Model file for the job. Use its own axes, mm. A direction names the side the tool comes from. Round coordinates to 2 decimals unless told otherwise and drop trailing zeros. Loops run counter-clockwise (first coordinate to the right, second up) from the corner with the lowest first, then second, coordinate; pieces in that order, holes last.
from build123d import *

# Parameters (mm, degrees)
SKETCH2_W                = 20
SKETCH2_H                = 64
BOSS_EXTRUDE1_DEPTH      = 30
SKETCH3_R                = 4
CUT_EXTRUDE1_DEPTH       = 20
SKETCH4_R                = 2.5
CUT_EXTRUDE2_DEPTH       = 10
FILLET1_R                = 10
BOSS_EXTRUDE2_DEPTH      = 20
BOSS_EXTRUDE2_DEPTH_BACK = 30
SKETCH5_W                = 2
SKETCH5_H                = 30
CUT_EXTRUDE3_REACH       = 55.161
SKETCH6_R                = 2.5
SKETCH6_W                = 10
SKETCH6_H                = 20
SKETCH6_W_2              = 20
SKETCH6_H_2              = 10
FILLET2_R                = 5
SKETCH7_W                = 21
SKETCH7_H                = 6
CUT_EXTRUDE4_DEPTH       = 10


with BuildPart() as part:
    # Sketch2 → Boss-Extrude1 (new body)
    with BuildSketch(Plane(origin=(0, 0, 0), x_dir=(1, 0, 0), z_dir=(0, 1, 0))):
        with Locations((6.47761194, -8.23880597)):
            Rectangle(SKETCH2_W, SKETCH2_H)
    extrude(amount=BOSS_EXTRUDE1_DEPTH)

    # Sketch3 → Cut-Extrude1 (cut)
    with BuildSketch(Plane(origin=(0, 30, 0), x_dir=(1, 0, 0), z_dir=(0, 1, 0))):
        with Locations(Location((6.47761194, 13.76119403, 0), (0, 0, 270))):
            Circle(SKETCH3_R)
        with Locations(Location((6.47761194, -30.23880597, 0), (0, 0, 270))):
            Circle(SKETCH3_R)
    extrude(amount=-CUT_EXTRUDE1_DEPTH, mode=Mode.SUBTRACT)

    # Sketch4 → Cut-Extrude2 (cut)
    with BuildSketch(Plane.ZY.offset(3.52238806)):
        with BuildLine():
            Line((17.415034126, 30.126407987), (14.795699792, 30.126407987))
            Line((14.795699792, 30.126407987), (14.949961333, 28.969446425))
            ThreePointArc((14.949961333, 28.969446425), (16.17927412, 22.186618473), (17.347611009, 28.980215007))
            Line((17.347611009, 28.980215007), (17.415034126, 30.126407987))
        make_face()
        with Locations((16.163554702, 25.686583173)):
            Circle(SKETCH4_R, mode=Mode.SUBTRACT)
    extrude(amount=-CUT_EXTRUDE2_DEPTH, mode=Mode.SUBTRACT)

    # Fillet1
    fillet1_edges = [part.edges().sort_by_distance(p)[0] for p in [
        (-3.52238806, 15, -23.76119403),
        (16.47761194, 15, -23.76119403),
        (16.47761194, 15, 40.23880597),
        (-3.52238806, 15, 40.23880597),
    ]]
    fillet(fillet1_edges, radius=FILLET1_R - 0.0001)  # a hair under: the kernel refuses the full size

    # Sketch5 → Boss-Extrude2 (add, two sides: drawn at the far end of the back side and taken through both)
    with BuildSketch(Plane.ZY.offset(3.52238806).offset(-BOSS_EXTRUDE2_DEPTH_BACK)):
        with Locations((6.23880597, 15)):
            Rectangle(SKETCH5_W, SKETCH5_H)
    extrude(amount=BOSS_EXTRUDE2_DEPTH + BOSS_EXTRUDE2_DEPTH_BACK)

    # Sketch6 → Cut-Extrude3 (cut, up to next)
    with BuildSketch(Plane(origin=(0, 0, 5.23880597), x_dir=(-1, 0, 0), z_dir=(0, 0, -1)), mode=Mode.PRIVATE) as cut_extrude3_sk1:
        with Locations((-21.47761194, 5)):
            Circle(SKETCH6_R)
    cut_extrude3_tool1 = extrude(cut_extrude3_sk1.sketch, amount=-CUT_EXTRUDE3_REACH, mode=Mode.PRIVATE) & part.part
    # Sketch6 → Cut-Extrude3 (cut, up to next)
    with BuildSketch(Plane(origin=(0, 0, 5.23880597), x_dir=(-1, 0, 0), z_dir=(0, 0, -1)), mode=Mode.PRIVATE) as cut_extrude3_sk2:
        with Locations((13.52238806, 5)):
            Circle(SKETCH6_R)
    cut_extrude3_tool2 = extrude(cut_extrude3_sk2.sketch, amount=-CUT_EXTRUDE3_REACH, mode=Mode.PRIVATE) & part.part
    # Sketch6 → Cut-Extrude3 (cut, up to next)
    with BuildSketch(Plane(origin=(0, 0, 5.23880597), x_dir=(-1, 0, 0), z_dir=(0, 0, -1)), mode=Mode.PRIVATE) as cut_extrude3_sk3:
        with Locations((-21.47761194, 20)):
            Rectangle(SKETCH6_W, SKETCH6_H)
    cut_extrude3_tool3 = extrude(cut_extrude3_sk3.sketch, amount=-CUT_EXTRUDE3_REACH, mode=Mode.PRIVATE) & part.part
    # Sketch6 → Cut-Extrude3 (cut, up to next)
    with BuildSketch(Plane(origin=(0, 0, 5.23880597), x_dir=(-1, 0, 0), z_dir=(0, 0, -1)), mode=Mode.PRIVATE) as cut_extrude3_sk4:
        with Locations((13.52238806, 25)):
            Rectangle(SKETCH6_W_2, SKETCH6_H_2)
    cut_extrude3_tool4 = extrude(cut_extrude3_sk4.sketch, amount=-CUT_EXTRUDE3_REACH, mode=Mode.PRIVATE) & part.part
    add(cut_extrude3_tool1.solids().sort_by_distance((21.477612, 5, 5.238806))[0], mode=Mode.SUBTRACT)
    add(cut_extrude3_tool2.solids().sort_by_distance((-13.522388, 5, 5.238806))[0], mode=Mode.SUBTRACT)
    add(cut_extrude3_tool3.solids().sort_by_distance((21.477612, 20, 5.238806))[0], mode=Mode.SUBTRACT)
    add(cut_extrude3_tool4.solids().sort_by_distance((-13.522388, 25, 5.238806))[0], mode=Mode.SUBTRACT)

    # Fillet2
    fillet2_edges = [part.edges().sort_by_distance(p)[0] for p in [
        (-23.52238806, 20, 6.23880597),
        (-23.52238806, 0, 6.23880597),
        (26.47761194, 0, 6.23880597),
        (26.47761194, 10, 6.23880597),
    ]]
    fillet(fillet2_edges, radius=FILLET2_R - 0.0001)  # a hair under: the kernel refuses the full size

    # Sketch7 → Cut-Extrude4 (cut)
    with BuildSketch(Plane(origin=(0, 0, 0), x_dir=(-1, 0, 0), z_dir=(0, -1, 0))):
        with Locations((-6.47761194, -10.23880597)):
            Rectangle(SKETCH7_W, SKETCH7_H)
    extrude(amount=-CUT_EXTRUDE4_DEPTH, mode=Mode.SUBTRACT)


solid = part.part
Q1. Flat gauge pins, fed straight in: P1, Ø6.5, axis at x = 6.48, z = 30.24, coming from the +Y side; P2, Ø2, axis at y = 6, z = 14, coming from the -X side; P3, Ø8, axis at x = 23.5, y = 4.5, coming from the -Z side. Where does each tip first touch, or does it go through?
Q2. Slice it at B-B on x = -1. Give the cut face in (y, z).
Q3. Probe line 1 (Z direction, x = 8.5, y = 23.25); line 2 (Z direction, x = 4, y = 26.75); line 3 (Z direction, x = 5.5, y = 21.75). List the from-to ranges inside material, lowest first.
Q4. Pull direction Z, two halves, no side cores. Call faces 5 (the face through (18, 5, 5.239)), 6 (the face through (-4, 8, 7.239)), 7 (the face through (-0.7, 15.2, 37.2)): pulls with the +Z half, pulls with the -Z half, needs draft (parallel to the pull), parting line crosses it, or undercut.
Q5. Slice it at A-A on y = 3.5. State how many separate pieces and enclosed holes the cut face has, plus the area to 3 significant figures.
Q6. Tool access for faces 1 (the face through (19, 10, 6)), 2 (the face through (-13, 10, 5.239)), 3 (the face through (7.679, 20.14, 34.054)), 4 (the face through (1.4, 27.8, 17.5)): list every direction of +Z, -Z, +X, -X, +Y, -Y with a clear straight run to the whole face (end or side of a thin tool).
Q7. Slice it at D-D on x = 20.5. Give the cut face in (y, z).
Reply:
1. P1: stops at y = 10
1. P2: stops at x = -3.52
1. P3: stops at z = 5.24
2. outline: (0, -20.4) - (30, -20.4) - (30, 14.81) - (28.97, 14.95) arc R3.5 cw (long way) to (28.98, 17.35) - (30, 17.41) - (30, 36.88) - (0, 36.88) - (0, 13.24) - (10, 13.24) - (10, 7.24) - (0, 7.24) - close; circle Ø5 at (25.69, 16.16)
3. line 1: z = -23.55 to -17.21, -10.31 to 26.79, 33.69 to 40.03
3. line 2: z = -23.45 to -16.9, -10.62 to 12.83, 13.9 to 18.43, 19.5 to 27.1, 33.38 to 39.93
3. line 3: z = -23.71 to -17.64, -9.88 to 26.36, 34.12 to 40.19
4. face 5: pulls with the -Z half
4. face 6: undercut
4. face 7: pulls with the +Z half
5. separate pieces: 4
5. enclosed holes: 0
5. area: 1,120 mm2
6. face 1: +Z, -Z, +X, +Y
6. face 2: -Z, -X, +Y, -Y
6. face 3: +Y
6. face 4: -X
7. outline: (0, 5.24) - (2.7, 5.24) - (2.7, 7.24) - (0, 7.24) - close; (7.3, 5.24) - (10, 5.24) - (10, 7.24) - (7.3, 7.24) - close
